Job drawing, mm, ordinate dimensions from the low corner. One solid piece. Coordinates: 2 decimals unless noted, no trailing zeros. Order: outer loops, then holes, each group sorted by start corner. A loop starts at its lowest first (then second) coordinate and runs counter-clockwise, first axis right, second up. Notation, with made-up numbers: (22.25, 14) - (43.25, 14) arc R21 cw to (43.25, 20) - close; hole circle Ø3 at (45.5, 1.25). An arc over 180 degrees is marked (long way). Return JSON: item names as keys, results as strings.
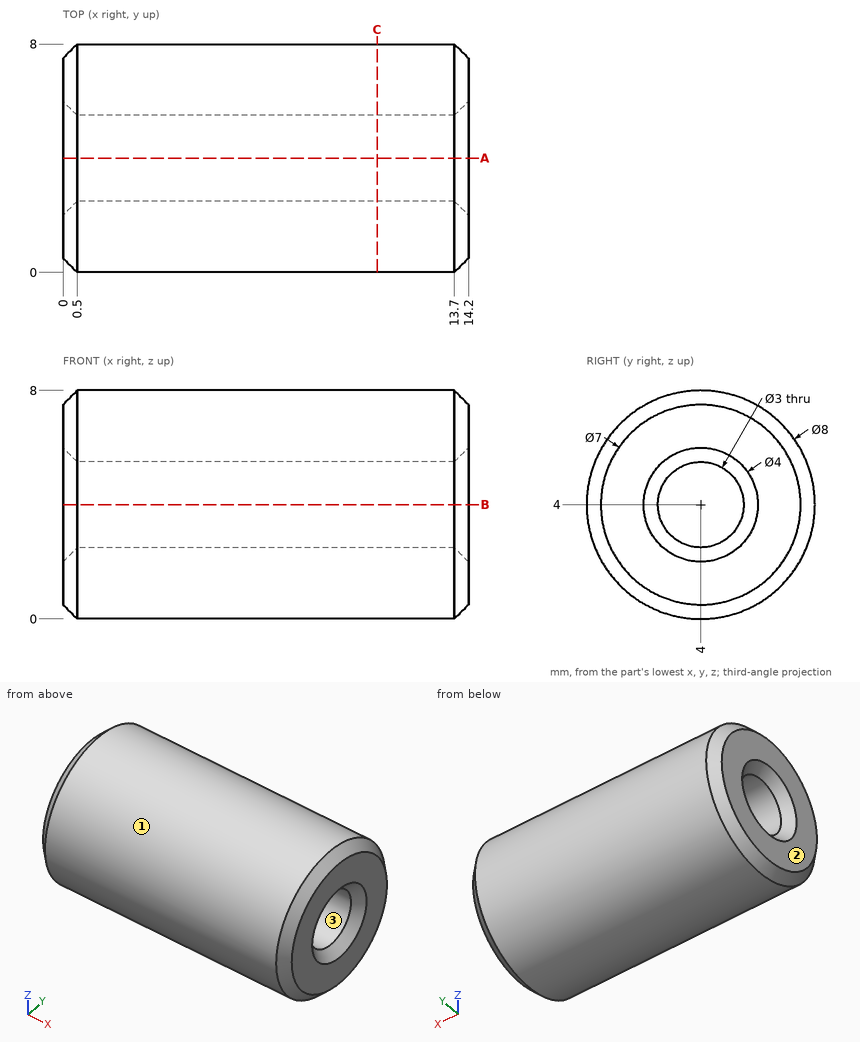
1. Probe L1, parallel to Z at x = 6.25, y = 4; L2, parallel to Y at x = 6.5, z = 4.25; L3, parallel to Y at x = 1.75, z = 2.75. List the from-to ranges inside material, lowest first.
Check values:
{"L1": "0 to 2.5, 5.5 to 8", "L2": "0.01 to 2.52, 5.48 to 7.99", "L3": "0.2 to 3.17, 4.83 to 7.8"}
2. Cut at C-C on x = 11. Give the cut face in (y, z), plus the area to 3 significant figures.
Check values:
{"outline": "circle Ø8 at (4, 4); hole circle Ø3 at (4, 4)", "area": "43.2 mm²"}
3. Mould opens along Z. For the marked faces 1, 2 and 3 say: pulls with the +Z half, pulls with the -Z half, needs draft (parallel to the pull), parting line crosses it, or undercut.
Check values:
{"face 1": "parting line crosses it", "face 2": "needs draft", "face 3": "undercut"}
4. Drop a flat-ended pin along its axis: pin 1 (4 mm diameter, centred on x = 1.5, z = 6.5, fed in from -Y). Give the stop position or say it passes through.
Check values:
{"pin 1": "y = 0.03"}
5. Cut at A-A on y = 4. Give the cut face in (x, z).
Check values:
{"outline": "(0, 0.5) - (0.5, 0) - (13.7, 0) - (14.2, 0.5) - (14.2, 2) - (13.7, 2.5) - (0.5, 2.5) - (0, 2) - close; (0, 6) - (0.5, 5.5) - (13.7, 5.5) - (14.2, 6) - (14.2, 7.5) - (13.7, 8) - (0.5, 8) - (0, 7.5) - close"}
